Read the model definition and answer for the solid it produces. Units are mm, in the model's axes. A direction names the side the tool comes from. Give positions to 0.01 mm unless a question says otherwise; leave off trailing zeros. Loops run counter-clockwise (first coordinate to the right, second up) from the corner with the lowest first, then second, coordinate; pieces in that order, holes last. Notation, with made-up numbers: M 68,85 L 126,85 A11 ccw 126,93 Z; hole C 75,-11 d6. An arc over 180 degrees is marked long. Return JSON: item names as keys, results as strings. Group by question number.
```python
from build123d import *

# Parameters (mm, degrees)
BOSS_EXTRUDE1_DEPTH = 36
SKETCH2_R           = 18
BOSS_EXTRUDE2_DEPTH = 20
BOSS_EXTRUDE3_START = 3
BOSS_EXTRUDE3_DEPTH = 4
HOLE1_D             = 24
CHAMFER1_SIZE       = 1
CUT_EXTRUDE1_DEPTH  = 87.116200566
FILLET1_R           = 8
HOLE2_D             = 8


with BuildPart() as part:
    # Sketch1 → Boss-Extrude1 (new body)
    with BuildSketch(Plane.XY):
        Polygon((0, 30), (0, 0), (66, 0), (66, 6), (6, 6), (6, 30), align=None)
    extrude(amount=BOSS_EXTRUDE1_DEPTH)

    # Sketch2 → Boss-Extrude2 (add)
    with BuildSketch(Plane(origin=(6, 0, 0), x_dir=(0, 0, -1), z_dir=(1, 0, 0))):
        with Locations(Location((-18, 30, 0), (0, 0, 90))):
            Circle(SKETCH2_R)
    extrude(amount=-BOSS_EXTRUDE2_DEPTH)

    # Sketch3 → Boss-Extrude3 (add)
    with BuildSketch(Plane.XY.offset(BOSS_EXTRUDE3_START)):
        Polygon((6, 25), (24, 6), (6, 6), align=None)
    boss_extrude3 = extrude(amount=BOSS_EXTRUDE3_DEPTH)

    # Mirror1: Boss-Extrude3 across plane
    add(boss_extrude3.mirror(Plane.XY.offset(18)))

    # Hole1 (through all)
    with Locations(Plane.ZY.offset(14)):
        with Locations((18, 30)):
            Hole(HOLE1_D / 2)

    # Chamfer1
    # the kernel refuses this chamfer: 1 mm, written as the material it takes off along each edge
    with BuildSketch(Plane(origin=(-14, 30, 18), x_dir=(0, 0, -1), z_dir=(0, -1, 0))) as chamfer1_piece_1:
        Polygon((12, CHAMFER1_SIZE), (12 + CHAMFER1_SIZE, 0), (12, 0), align=None)
    revolve(axis=Axis((-14, 30, 18), (1, 0, 0)), mode=Mode.SUBTRACT)
    with BuildSketch(Plane(origin=(6, 30, 18), x_dir=(0, 0, -1), z_dir=(0, -1, 0))) as chamfer1_piece_2_section:
        Polygon((12 + CHAMFER1_SIZE, 0), (12, -CHAMFER1_SIZE), (12, 0), align=None)
    chamfer1_piece_2 = revolve(axis=Axis((6, 30, 18), (1, 0, 0)), mode=Mode.PRIVATE)
    chamfer1_piece_2 = split(chamfer1_piece_2, bisect_by=Plane(origin=(1.543769163, 29.703799217, 6.002209696), z_dir=(0.7259526839058266, 0.6877446479107833, 0)), keep=Keep.TOP, mode=Mode.PRIVATE)
    add(chamfer1_piece_2, mode=Mode.SUBTRACT)
    with BuildSketch(Plane(origin=(6, 30, 18), x_dir=(0, 0, -1), z_dir=(0, -1, 0))) as chamfer1_piece_3_section:
        Polygon((12 + CHAMFER1_SIZE, 0), (12, -CHAMFER1_SIZE), (12, 0), align=None)
    chamfer1_piece_3 = revolve(axis=Axis((6, 30, 18), (1, 0, 0)), mode=Mode.PRIVATE)
    chamfer1_piece_3 = split(chamfer1_piece_3, bisect_by=Plane(origin=(5.516878747, 17.516878747, 7), z_dir=(0, 0, 1)), keep=Keep.TOP, mode=Mode.PRIVATE)
    chamfer1_piece_3 = split(chamfer1_piece_3, bisect_by=Plane(origin=(5.516878747, 17.516878747, 29), z_dir=(0, 0, -1)), keep=Keep.TOP, mode=Mode.PRIVATE)
    add(chamfer1_piece_3, mode=Mode.SUBTRACT)

    # Sketch7 → Cut-Extrude1 (cut, through all)
    with BuildSketch(Plane(origin=(0, 6, 0), x_dir=(1, 0, 0), z_dir=(0, 1, 0))):
        with BuildLine():
            Line((31, -10), (39, -10))
            ThreePointArc((39, -10), (47, -18), (39, -26))
            Line((39, -26), (31, -26))
            ThreePointArc((31, -26), (23, -18), (31, -10))
        make_face()
    extrude(amount=-CUT_EXTRUDE1_DEPTH, mode=Mode.SUBTRACT)

    # Fillet1
    fillet1_edges = [part.edges().sort_by_distance(p)[0] for p in [
        (66, 3, 36),
        (66, 3, 0),
    ]]
    fillet(fillet1_edges, radius=FILLET1_R)

    # Hole2 (through all)
    with Locations(Plane(origin=(0, 6, 0), x_dir=(1, 0, 0), z_dir=(0, 1, 0))):
        with Locations((58, -8), (58, -28)):
            Hole(HOLE2_D / 2)


solid = part.part
```
1. Find section B-B (x = 13.5). Write down the section's boundary in (y, z), and give its area (3 significant figures).
2. Find section D-D (y = 44.5). Write down the section's boundary in (x, z), and give its area (3 significant figures).
3. Find section C-C (z = 16). State how many separate pieces and enclosed holes the cut face has, and give its area (3 significant figures).
4. Flat-ended cylindrical pins translate along their axes: P1, Ø9, axis at y = 19, z = 18.5, coming from the -X side; P2, Ø13.5, axis at y = 16, z = 16, coming from the +X side; P3, Ø6, axis at y = 25.5, z = 6.5, coming from the +X side; P4, Ø7, axis at x = 58, z = 28, coming from the -Y side. Find the tip coordinate at first contact, or state that the pin passes through.
5. The mould has two halves that part along Z. Classify faces 1 (the flat face through (10, 14, 7)), 2 (the flat face through (18, 5, 36)), 3 (the flat face through (32.5, 0, 9.7)): +Z half, -Z half, draft (parallel to the pull), parting line (faces both ways), or undercut.
6. Straight lines are drawn through the part: line 1 along X through (y, z) = (1.7, 28); line 2 along Z through (x, y) = (-2, 30); line 3 along Z through (x, y) = (58, 1). For each, find the intervals that lie inside material, in ascending order.
7. For faces 4 (the flat face through (66, 3, 18)), 5 (the flat face through (-14, 39.2, 27.4)), 6 (the flat face through (6, 13, 18)), 7 (the conical face through (5.2, 17.8, 18.2)), 8 (the cylindrical face through (47, 3, 18)), determine the directions among +Z, -Z, +X, -X, +Y, -Y from which every point of the face is accessible in a straight line to the end or side of a thin tool.
8. Find section A-A (x = 55.5). Write down the section's boundary in (y, z), and give its area (3 significant figures).
Result:
{
 "1": {"outline": "M 0,0 L 6,0 L 6,3 L 17.08,3 L 17.08,7 L 6,7 L 6,29 L 17.08,29 L 17.08,33 L 6,33 L 6,36 L 0,36 Z", "area": "305 mm2"},
 "2": {"outline": "M -14,7.33 L 6,7.33 L 6,28.67 L -14,28.67 Z", "area": "427 mm2"},
 "3": {"separate pieces": "3", "enclosed holes": "0", "area": "532 mm2"},
 "4": {"P1": "stops at x = -14", "P2": "stops at x = 6", "P3": "stops at x = 8.37", "P4": "passes through"},
 "5": {"face 1": "undercut", "face 2": "+Z half", "face 3": "draft"},
 "6": {"line 1": "x = 0 to 54, 62 to 66", "line 2": "z = 0 to 6, 30 to 36", "line 3": "z = 0 to 4, 12 to 24, 32 to 36"},
 "7": {"face 4": "+Z, -Z, +X, +Y, -Y", "face 5": "+Z, -Z, -X, +Y, -Y", "face 6": "+X, +Y", "face 7": "+X", "face 8": "+Y, -Y"},
 "8": {"outline": "M 0,0 L 6,0 L 6,4.88 L 0,4.88 Z; M 0,11.12 L 6,11.12 L 6,24.88 L 0,24.88 Z; M 0,31.12 L 6,31.12 L 6,36 L 0,36 Z", "area": "141 mm2"}
}
